Source: CAD feature listing. Evaluate the final solid. Frame: model axes, mm. Round coordinates to 2 decimals unless told otherwise and drop trailing zeros. Loops run counter-clockwise (first coordinate to the right, second up) from the corner with the lowest first, then second, coordinate; pieces in that order, holes last. Notation, with made-up numbers: (67, 78.5) -> (75, 78.5) arc R22 ccw to (75, 86.5) -> close; hole circle Ø7 at (43.5, 73.5). An arc over 180 degrees is marked (long way). Write item = value, one per line.
from build123d import *

# Parameters (mm, degrees)
F0_W     = 50.8
F0_H     = 50.8
F0_R     = 3.175
F1_DEPTH = 12.7
F2_DEPTH = 31.75
F3_DEPTH = 19.05


with BuildPart() as f1:
    # F0 (on Top) → F1 (new body)
    with BuildSketch(Plane.XY):
        Polygon((0, 304.8), (0, 0), (320.675, 0), (320.675, 45.903602), (214.3506, 152.339401), (320.675, 258.7752), (320.675, 304.8), align=None)
        with Locations((73.025, 152.4)):
            Rectangle(F0_W, F0_H, mode=Mode.SUBTRACT)
        with Locations((73.025, 152.4)):
            Rectangle(F0_W, F0_H)
        with Locations((73.025, 152.4)):
            Circle(F0_R, mode=Mode.SUBTRACT)
    extrude(amount=F1_DEPTH)

    # F0 (on Top) → F2 (join)
    with BuildSketch(Plane.XY):
        with Locations((73.025, 152.4)):
            Rectangle(F0_W, F0_H)
        with Locations((73.025, 152.4)):
            Circle(F0_R, mode=Mode.SUBTRACT)
    extrude(amount=F2_DEPTH)

    # F0 (on Top) → F3 (join)
    with BuildSketch(Plane.XY):
        with Locations((73.025, 152.4)):
            Rectangle(F0_W, F0_H)
        with Locations((73.025, 152.4)):
            Circle(F0_R, mode=Mode.SUBTRACT)
    extrude(amount=-F3_DEPTH)


solid = f1.part
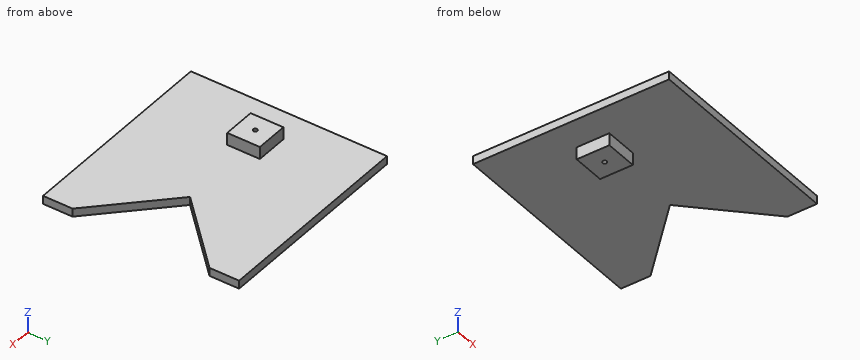
1. Section query D-D (x = 284.5). Return the cut outline in (y, z), then the cut area to 3 significant figures.
Evaluation:
outline = (0, 0) -> (82.12, 0) -> (82.12, 12.7) -> (0, 12.7) -> close; (222.56, 0) -> (304.8, 0) -> (304.8, 12.7) -> (222.56, 12.7) -> close
area = 2,090 mm²
2. Section query C-C (y = 42). Return the cut outline in (x, z) (3 decimals).
Evaluation:
outline = (0, 0) -> (320.675, 0) -> (320.675, 12.7) -> (0, 12.7) -> close
3. Contact query for flat-ended pins moving along their axis: pin 1 Ø9.5 at (y, z) = (156, -5.5) entering from -X (3 decimals); pin 2 Ø10 at (x, y) = (219.5, 81) entering from +Z; pin 3 Ø21 at (x, z) = (66, -12) entering from -Y; pin 4 Ø4 at (x, y) = (73.025, 152.4) entering from -Z. Output: stop coordinate, or through.
Evaluation:
pin_1 = 47.625
pin_2 = 12.7
pin_3 = 127
pin_4 = through
4. Line query: probe 1 along X at (y, z) = (152.4, -13) (3 decimals); probe 2 along X at (y, z) = (152.4, 10); probe 3 along X at (y, z) = (167, -9.5) (3 decimals). Output: solid intervals per line, ascending. Write a range as from..to.
Evaluation:
probe_1 = 47.625..69.85, 76.2..98.425
probe_2 = 0..69.85, 76.2..214.41
probe_3 = 47.625..98.425
5. Section query A-A (x = 236). Return the cut outline in (y, z).
Evaluation:
outline = (0, 0) -> (130.67, 0) -> (130.67, 12.7) -> (0, 12.7) -> close; (174.01, 0) -> (304.8, 0) -> (304.8, 12.7) -> (174.01, 12.7) -> close
6. Section query B-B (z = -9). Return the cut outline in (x, y) (3 decimals).
Evaluation:
outline = (47.625, 127) -> (98.425, 127) -> (98.425, 177.8) -> (47.625, 177.8) -> close; hole circle Ø6.35 at (73.025, 152.4)
